Input: part model. Units: mm. Frame: model coordinates. Face numbers are marked on the shaded views. A direction names the side the tool comes from. Give positions to 0.01 mm unless a question says otherwise; leave off trailing zeros. Loops run counter-clockwise (first coordinate to the right, second up) from the corner with the lowest first, then second, coordinate; pieces in that order, holes last. Notation, with made-up numbers: M -1,88 L 31,88 A14 ccw 31,110 Z; hole C 78,62 d3. An arc over 180 degrees is marked long. Use a Markdown table: item, result. Add a question column.
Autodesk Inventor part; units mm, degrees
ref_plane "YZ Plane" through (0, 0, 0) normal (1, 0, 0) x (0, 1, 0)
ref_plane "XZ Plane" through (0, 0, 0) normal (0, 1, 0) x (-1, 0, 0)
ref_plane "XY Plane" through (0, 0, 0) normal (0, 0, 1) x (1, 0, 0)
sketch "Sketch1" plane through (0, 0, 0) normal (0, 0, 1) x (1, 0, 0)
  line L0 (0, 23.5) -> (9.3, 23.5)
  line L1 (9.7, 23.9) -> (9.7, 29.2)
  line L2 (9.7, 29.2) -> (16.1, 29.2)
  line L3 (16.1, 29.2) -> (16.1, 31.5)
  line L4 (16.1, 31.5) -> (0, 31.5)
  line L5 (0, 23.5) -> (0, 39.7331)
  arc A0 (9.3, 23.5) -> (9.7, 23.9) centre (9.3, 23.9) ccw
  line L6 (0, 0) -> (48.7382, 0)
  line L7 (0, 23.5) -> (-9.3, 23.5)
  line L8 (-9.7, 23.9) -> (-9.7, 29.2)
  line L9 (-9.7, 29.2) -> (-16.1, 29.2)
  line L10 (-16.1, 29.2) -> (-16.1, 31.5)
  line L11 (-16.1, 31.5) -> (0, 31.5)
  arc A1 (-9.7, 23.9) -> (-9.3, 23.5) centre (-9.3, 23.9) ccw
  dimension "d0" = 0.4
  dimension "d1" = 47
  dimension "d2" = 63
  dimension "d3" = 58.4
  dimension "d4" = 16.1
  dimension "d5" = 9.7
revolve "Revolution1" add sketch "Sketch1" angle 360 about axis through (0, 0, 0) along (1, 0, 0)
properties part number "3136 7009 52" material "Nylon 6/6"
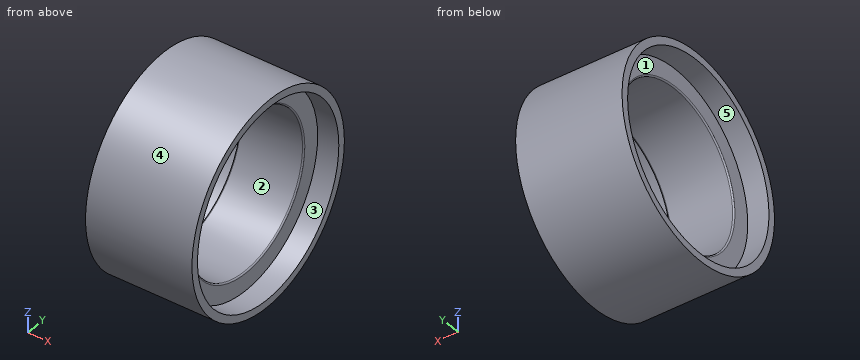
1) Contact query for flat-ended pins moving along their axis: P1, Ø6, axis at x = 6.5, z = 14, coming from the +Y side; P2, Ø2, axis at x = 9.5, y = 2.5, coming from the -Z side; P3, Ø2, axis at x = -5, z = 20, coming from the +Y side. Output: stop coordinate, or through.
2) Section query D-D, the plane z = 25. Return the cut outline in (x, y).
3) Pull-direction query (Z, two-part tool) for the marked faces 4 and 5; classes: pulls with the +Z half, pulls with the -Z half, needs draft (parallel to the pull), parting line crosses it, or undercut.
4) Section query A-A, the plane z = 0. Return the cut outline in (x, y).
5) Reachability of the marked faces 1, 2 and 3 from +Z, -Z, +X, -X, +Y, -Y: full face, straight path, thin tool, end or side. Return the list, or none.
6) Section query C-C, the plane x = -1. Return the cut outline in (y, z), and give its area (3 significant figures).
7) Ray query, line 1 (Y direction, x = 0, z = -0.5); line 2 (Z direction, x = 0.25, y = 0); line 3 (X direction, y = 17.5, z = 20). Return the intervals inside material, ascending. Write a range as [from, to].
Entries:
| question | item | result |
|---|---|---|
| 1 | P1 | stops at y = 29.52 |
| 1 | P2 | stops at z = -31.46 |
| 1 | P3 | stops at y = 25.12 |
| 2 | outline | M -16.1,-19.16 L 16.1,-19.16 L 16.1,-15.09 L 9.7,-15.09 L 9.7,15.09 L 16.1,15.09 L 16.1,19.16 L -16.1,19.16 L -16.1,15.09 L -9.7,15.09 L -9.7,-15.09 L -16.1,-15.09 Z |
| 3 | face 4 | parting line crosses it |
| 3 | face 5 | undercut |
| 4 | outline | M -16.1,-31.5 L 16.1,-31.5 L 16.1,-29.2 L 9.7,-29.2 L 9.7,-23.9 A0.4 ccw 9.3,-23.5 L -9.3,-23.5 A0.4 ccw -9.7,-23.9 L -9.7,-29.2 L -16.1,-29.2 Z; M -16.1,29.2 L -9.7,29.2 L -9.7,23.9 A0.4 ccw -9.3,23.5 L 9.3,23.5 A0.4 ccw 9.7,23.9 L 9.7,29.2 L 16.1,29.2 L 16.1,31.5 L -16.1,31.5 Z |
| 5 | face 1 | -X |
| 5 | face 2 | +X, -X |
| 5 | face 3 | +X |
| 6 | outline | C 0,0 d63; hole C 0,0 d47 |
| 6 | area | 1,380 mm² |
| 7 | line 1 | y = [-31.5, -23.49], [23.49, 31.5] |
| 7 | line 2 | z = [-31.5, -23.5], [23.5, 31.5] |
| 7 | line 3 | x = [-9.7, 9.7] |
